Could you check a few things on this drawing? It's one solid part, dimensions in mm from its lowest x, y, z. A direction names the side the tool comes from. Give positions to 0.01 mm unless a question says otherwise; leave off trailing zeros. Loops run counter-clockwise (first coordinate to the right, second up) from the corner with the lowest first, then second, coordinate; pieces in that order, holes last. Notation, with made-up numbers: (-8, 77.25) - (14, 77.25) arc R20 cw to (14, 112.25) - close; hole circle Ø10 at (39, 17.25). An arc over 180 degrees is marked (long way). Put each result on its own line as item: value. Start each with the question number.
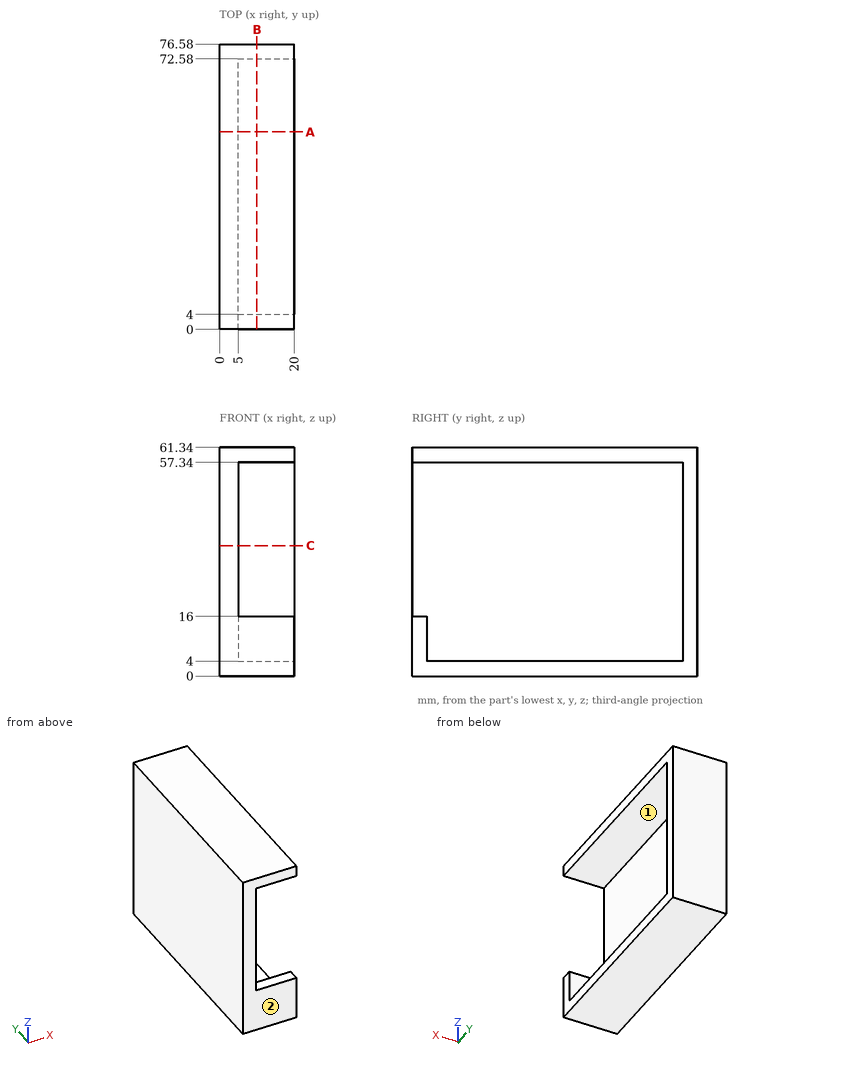
1) I'm going to push flat-ended pins straight in: P1, Ø4.5, axis at x = 10, z = 23.5, coming from the -Y side; P2, Ø10, axis at y = 65, z = 49.5, coming from the +X side. Where does each tip first touch, or does it pass through?
2) Suppose I cut it at C-C on z = 35. Please give me the cut outline in (x, y), plus the area to 3 significant figures.
3) I need wall thicknesses on line 1 (Y direction, x = 15, z = 15); line 2 (Z direction, x = 14, y = 39); line 3 (Z direction, x = 14.75, y = 3). Which ranges of each line are inside material? Lowest first, please.
4) Suppose I cut it at A-A on y = 53. Please give me the cut outline in (x, z), plus the area to 3 significant figures.
5) Suppose I cut it at B-B on x = 10. Please give me the cut outline in (y, z).
6) Which directions (+Z, -Z, +X, -X, +Y, -Y) give clear straight access to the entire face, cutting with the end or side of a thin tool? Please do the marked faces 1 and 2.
Ans:
1. P1: stops at y = 72.58
1. P2: stops at x = 5
2. outline: (0, 0) - (5, 0) - (5, 72.58) - (20, 72.58) - (20, 76.58) - (0, 76.58) - close
2. area: 443 mm²
3. line 1: y = 0 to 4, 72.58 to 76.58
3. line 2: z = 0 to 4, 57.34 to 61.34
3. line 3: z = 0 to 16, 57.34 to 61.34
4. outline: (0, 0) - (20, 0) - (20, 4) - (5, 4) - (5, 57.34) - (20, 57.34) - (20, 61.34) - (0, 61.34) - close
4. area: 427 mm²
5. outline: (0, 0) - (76.58, 0) - (76.58, 61.34) - (0, 61.34) - (0, 57.34) - (72.58, 57.34) - (72.58, 4) - (4, 4) - (4, 16) - (0, 16) - close
6. face 1: +X, -Y
6. face 2: +Z, -Z, +X, -X, -Y
